Here's how the part is built. I have some questions about the finished solid (model axes, mm). A direction names the side the tool comes from. Round coordinates to 2 decimals unless told otherwise and drop trailing zeros. Order: outer loops, then holes, each group sorted by start corner. A loop starts at its lowest first (then second) coordinate and runs counter-clockwise, first axis right, second up. Notation, with made-up numbers: M 60,-9 L 92,-9 A32 cw 92,28 Z; hole C -2,-14.75 d11. An arc over 180 degrees is marked long. Write item = value, one per line. Start each with the question number.
Item 1: I'm going to push flat-ended pins straight in: P1, Ø1.9, axis at x = 80, y = 12.8, coming from the +Z side; P2, Ø8, axis at y = 20, z = 4, coming from the +X side; P3, Ø5, axis at x = 0, z = -13.5, coming from the +Y side; P4, Ø12, axis at y = 43.5, z = -25, coming from the -X side. Where does each tip first touch, or does it pass through?
Item 2: Please list where these lines run through material, in increasing order: L1, parallel to X at y = 3, z = 6; L2, parallel to X at y = 3.3, z = -6.75; L3, parallel to X at y = 60, z = 4.
Item 3: I want a section at C-C, the plane x = 66. List the corners of the cut face in (y, z) for me.
Item 4: I want a section at A-A, the plane x = 91. List the corners of the cut face in (y, z) for me, plus the area to 3 significant figures.
Item 5: For faces 4 (the face through (42.465, 25.558, 10.372)), 5 (the face through (100.4, 49.3, -46.5)), 6 (the face through (45, 38, -10)), which set-ups out of +Z, -Z, +X, -X, +Y, -Y let a thin tool reach every point of the face, with its end or its side?
Item 6: We'd pull the mould along Y, two halves only. Please class faces 1 (the face through (108.493, 37.173, -46.465)), 2 (the face through (42.54, 24.51, -2.24)), 3 (the face through (-20, 2, 0)): pulls with the +Y half, pulls with the -Y half, needs draft (parallel to the pull), parting line crosses it, or undercut.
Item 7: I want a section at B-B, the plane y = 12.8. List the corners of the cut face in (x, z) for me.
```python
from build123d import *

# Parameters (mm, degrees)
EXTRUDE_1_DEPTH     = 5
SKETCH_3_R          = 1.6
CUT_EXTRUDE_1_DEPTH = 11
EXTRUDE_3_DEPTH     = 5
EXTRUDE_4_DEPTH     = 5
SKETCH_25_R         = 20
CUT_EXTRUDE_2_DEPTH = 5
FILLET_1_R          = 4
FILLET_4_R          = 9
SKETCH_19_R         = 7.5
CUT_EXTRUDE_3_DEPTH = 5
SKETCH_26_R         = 1.6
CUT_EXTRUDE_4_DEPTH = 5
FILLET_5_R          = 10
CUT_EXTRUDE_5_DEPTH = 5
FILLET_10_R         = 2
FILLET_11_R         = 3


with BuildPart() as part:
    # 草图1 → 凸台-拉伸1 (new body)
    with BuildSketch(Plane(origin=(0, 0, 0), x_dir=(1, 0, 0), z_dir=(0, 1, 0))):
        with BuildLine():
            Line((45, 20), (0, 20))
            ThreePointArc((0, 20), (-20, 0), (0, -20))
            Line((0, -20), (45, -20))
            Line((45, -20), (45, 20))
        make_face()
    extrude(amount=EXTRUDE_1_DEPTH)

    # 草图3 → 切除-拉伸1 (cut)
    with BuildSketch(Plane(origin=(0, 5, 0), x_dir=(1, 0, 0), z_dir=(0, 1, 0))):
        with Locations((0, 13.5)):
            Circle(SKETCH_3_R)
        with Locations((11.691342951, 6.75)):
            Circle(SKETCH_3_R)
        with Locations((11.691342951, -6.75)):
            Circle(SKETCH_3_R)
        with Locations((0, -13.5)):
            Circle(SKETCH_3_R)
        with Locations((-11.691342951, -6.75)):
            Circle(SKETCH_3_R)
        with Locations((-11.691342951, 6.75)):
            Circle(SKETCH_3_R)
    extrude(amount=-CUT_EXTRUDE_1_DEPTH, mode=Mode.SUBTRACT)

    # 草图22 → 凸台-拉伸3 (add)
    with BuildSketch(Plane(origin=(45, 0, 0), x_dir=(0, 0, -1), z_dir=(1, 0, 0))):
        Polygon((-20, 5), (20, 5), (20, 9.3), (44, 9.3), (44, 66.3), (-20, 66.3), align=None)
    extrude(amount=-EXTRUDE_3_DEPTH)

    # 草图24 → 凸台-拉伸4 (add)
    with BuildSketch(Plane(origin=(0, 0, -44), x_dir=(-1, 0, 0), z_dir=(0, 0, -1))):
        with BuildLine():
            Line((-40, 9.3), (-80, 9.3))
            ThreePointArc((-80, 9.3), (-108.5, 37.8), (-80, 66.3))
            Line((-80, 66.3), (-40, 66.3))
            Line((-40, 66.3), (-40, 9.3))
        make_face()
    extrude(amount=EXTRUDE_4_DEPTH)

    # 草图25 → 切除-拉伸2 (cut)
    with BuildSketch(Plane(origin=(0, 0, -49), x_dir=(-1, 0, 0), z_dir=(0, 0, -1))):
        with Locations((-80, 37.8)):
            Circle(SKETCH_25_R)
    extrude(amount=-CUT_EXTRUDE_2_DEPTH, mode=Mode.SUBTRACT)

    # 圆角1
    fillet_1_edges = [part.edges().sort_by_distance(p)[0] for p in [
        (40, 5, 0),
        (45, 37.8, -44),
    ]]
    fillet(fillet_1_edges, radius=FILLET_1_R)

    # 圆角4
    fillet_4_edges = [part.edges().sort_by_distance(p)[0] for p in [
        (45, 0, 0),
        (40, 37.8, -49),
    ]]
    fillet(fillet_4_edges, radius=FILLET_4_R)

    # 草图19 → 切除-拉伸3 (cut)
    with BuildSketch(Plane.XZ):
        Circle(SKETCH_19_R)
    extrude(amount=-CUT_EXTRUDE_3_DEPTH, mode=Mode.SUBTRACT)

    # 草图26 → 切除-拉伸4 (cut)
    with BuildSketch(Plane.XY.offset(-44)):
        with Locations((101.650635095, 50.3)):
            Circle(SKETCH_26_R)
        with Locations((101.650635095, 25.3)):
            Circle(SKETCH_26_R)
        with Locations((80, 12.8)):
            Circle(SKETCH_26_R)
        with Locations((58.349364905, 25.3)):
            Circle(SKETCH_26_R)
        with Locations((58.349364905, 50.3)):
            Circle(SKETCH_26_R)
        with Locations((80, 62.8)):
            Circle(SKETCH_26_R)
    extrude(amount=-CUT_EXTRUDE_4_DEPTH, mode=Mode.SUBTRACT)

    # 圆角5
    fillet_5_edges = [part.edges().sort_by_distance(p)[0] for p in [
        (42.5, 66.3, 20),
    ]]
    fillet(fillet_5_edges, radius=FILLET_5_R)

    # 草图27 → 切除-拉伸5 (cut)
    with BuildSketch(Plane(origin=(45, 0, 0), x_dir=(0, 0, -1), z_dir=(1, 0, 0))):
        Polygon((10.027417726, 43.207223614), (-7.542180321, 59.853257478), (27.457819679, 59.853257478), align=None)
        Polygon((15.84211595, 37.698181047), (31.611388693, 52.757836516), (31.611388693, 22.757836516), align=None)
        Polygon((-7.31927621, 15.272435239), (27.678973834, 15.622426489), (10.082987202, 32.093328411), align=None)
        Polygon((-11.611388693, 52.757836516), (-11.611388693, 22.757836516), (4.15788405, 37.698181047), align=None)
    extrude(amount=-CUT_EXTRUDE_5_DEPTH, mode=Mode.SUBTRACT)

    # 圆角10
    fillet_10_edges = [part.edges().sort_by_distance(p)[0] for p in [
        (42.5, 15.272435239, 7.31927621),
        (42.5, 15.622426489, -27.678973834),
        (42.5, 22.757836516, -31.611388693),
        (42.5, 52.757836516, -31.611388693),
        (42.5, 52.757836516, 11.611388693),
        (42.5, 22.757836516, 11.611388693),
        (42.5, 59.853257478, -27.457819679),
        (42.5, 59.853257478, 7.542180321),
    ]]
    fillet(fillet_10_edges, radius=FILLET_10_R)

    # 圆角11
    fillet_11_edges = [part.edges().sort_by_distance(p)[0] for p in [
        (42.5, 32.093328411, -10.082987202),
        (42.5, 37.698181047, -15.84211595),
        (42.5, 37.698181047, -4.15788405),
        (42.5, 43.207223614, -10.027417726),
    ]]
    fillet(fillet_11_edges, radius=FILLET_11_R)


solid = part.part
```
Filled in:
q1.P1 = through
q1.P2 = 45
q1.P3 = 5
q1.P4 = 40
q2.L1 = -19.08 to -13.1, -10.28 to -4.5, 4.5 to 10.28, 13.1 to 42.71
q2.L2 = -18.83 to -13.29, -10.09 to -3.27, 3.27 to 10.09, 13.29 to 42.96
q2.L3 = 40 to 45
q3.outline = M 9.3,-49 L 23.52,-49 L 23.52,-44 L 9.3,-44 Z; M 52.08,-49 L 66.3,-49 L 66.3,-44 L 52.08,-44 Z
q4.outline = M 11.51,-49 L 21.1,-49 L 21.1,-44 L 11.51,-44 Z; M 54.5,-49 L 64.09,-49 L 64.09,-44 L 54.5,-44 Z
q4.area = 95.9 mm^2
q5.face_4 = +X, -X
q5.face_5 = +Z, -Z
q5.face_6 = +Z, +X, +Y, -Y
q6.face_1 = parting line crosses it
q6.face_2 = undercut
q6.face_3 = needs draft
q7.outline = M 40,-40 A9 ccw 49,-49 L 78.4,-49 L 78.4,-44 L 49,-44 A4 cw 45,-40 L 45,20 L 40,20 Z; M 81.6,-49 L 93.68,-49 L 93.68,-44 L 81.6,-44 Z
